The listing builds one solid part. Answer for the finished solid, in the listing's coordinates (mm). A direction names the side the tool comes from. Round coordinates to 2 decimals unless told otherwise and drop trailing zeros. Order: outer loops, then holes, each group sorted by start corner. A loop starts at its lowest first (then second) coordinate and runs counter-clockwise, first axis right, second up. Notation, with made-up numbers: (5.25, 35.5) - (56.25, 35.5) arc R13 cw to (56.25, 41.5) - close; hole circle Ø7 at (-7.75, 84). An arc over 180 degrees is marked (long way). Write item = value, one per line.
from build123d import *

# Parameters (mm, degrees)
ESQUISSE1_W             = 136.8
ESQUISSE1_H             = 11.8
BOSS_EXTRU_1_DEPTH      = 0.8
ESQUISSE2_W             = 136.8
ESQUISSE2_H             = 11.8
ESQUISSE2_W_2           = 135.2
ESQUISSE2_H_2           = 10.2
BOSS_EXTRU_2_DEPTH      = 1
ESQUISSE3_W             = 4
ESQUISSE3_H             = 0.8
BOSS_EXTRU_3_DEPTH      = 2
ESQUISSE4_W             = 11.8
ESQUISSE4_H             = 0.8
BOSS_EXTRU_4_DEPTH      = 5
ESQUISSE5_W             = 11.8
ESQUISSE5_H             = 0.8
BOSS_EXTRU_5_DEPTH      = 5
ESQUISSE6_R             = 1.2
ENL_V_MAT_EXTRU_1_DEPTH = 4
CONG_1_R                = 1


with BuildPart() as part:
    # Esquisse1 → Boss.-Extru.1 (new body)
    with BuildSketch(Plane(origin=(0, 0, 0), x_dir=(1, 0, 0), z_dir=(0, 1, 0))):
        with Locations((68.4, 5.9)):
            Rectangle(ESQUISSE1_W, ESQUISSE1_H)
    extrude(amount=BOSS_EXTRU_1_DEPTH)

    # Esquisse2 → Boss.-Extru.2 (add)
    with BuildSketch(Plane(origin=(0, 0.8, 0), x_dir=(1, 0, 0), z_dir=(0, 1, 0))):
        with Locations((68.4, 5.9)):
            Rectangle(ESQUISSE2_W, ESQUISSE2_H)
        with Locations((68.4, 5.9)):
            Rectangle(ESQUISSE2_W_2, ESQUISSE2_H_2, mode=Mode.SUBTRACT)
    extrude(amount=BOSS_EXTRU_2_DEPTH)

    # Esquisse3 → Boss.-Extru.3 (add)
    with BuildSketch(Plane(origin=(0, 1.8, 0), x_dir=(1, 0, 0), z_dir=(0, 1, 0))):
        Polygon((0.8, 3), (0, 3), (0, 0), (3, 0), (3, 0.8), (0.8, 0.8), align=None)
        Polygon((3, 11.8), (0, 11.8), (0, 8.8), (0.8, 8.8), (0.8, 11), (3, 11), align=None)
        Polygon((133.8, 11), (136, 11), (136, 8.8), (136.8, 8.8), (136.8, 11.8), (133.8, 11.8), align=None)
        with Locations((68.4, 11.4)):
            Rectangle(ESQUISSE3_W, ESQUISSE3_H)
        with Locations((68.4, 0.4)):
            Rectangle(ESQUISSE3_W, ESQUISSE3_H)
        Polygon((133.8, 0), (136.8, 0), (136.8, 3), (136, 3), (136, 0.8), (133.8, 0.8), align=None)
    extrude(amount=BOSS_EXTRU_3_DEPTH)

    # Esquisse4 → Boss.-Extru.4 (add)
    with BuildSketch(Plane(origin=(136.8, 0, 0), x_dir=(0, 0, -1), z_dir=(1, 0, 0))):
        with Locations((5.9, 0.4)):
            Rectangle(ESQUISSE4_W, ESQUISSE4_H)
    extrude(amount=BOSS_EXTRU_4_DEPTH)

    # Esquisse5 → Boss.-Extru.5 (add)
    with BuildSketch(Plane.ZY):
        with Locations((-5.9, 0.4)):
            Rectangle(ESQUISSE5_W, ESQUISSE5_H)
    extrude(amount=BOSS_EXTRU_5_DEPTH)

    # Esquisse6 → Enlèv. mat.-Extru.1 (cut)
    with BuildSketch(Plane.XZ):
        with Locations((140, -5.9)):
            Circle(ESQUISSE6_R)
        with Locations((-3.2, -5.9)):
            Circle(ESQUISSE6_R)
    extrude(amount=-ENL_V_MAT_EXTRU_1_DEPTH, mode=Mode.SUBTRACT)

    # Congé1
    cong_1_edges = [part.edges().sort_by_distance(p)[0] for p in [
        (141.8, 0.4, -11.8),
        (141.8, 0.4, 0),
        (-5, 0.4, -11.8),
        (-5, 0.4, 0),
        (0, 2.3, -11.8),
        (136.8, 2.3, -11.8),
        (136.8, 2.3, 0),
        (0, 2.3, 0),
    ]]
    fillet(cong_1_edges, radius=CONG_1_R)


solid = part.part
Q1. Determine the mould class of faces 5 (the face through (139.4, 0.8, -4.5)), 6 (the face through (69, 1, 0)), 7 (the face through (69, 2, -0.8)), 8 (the face through (138.8, 0.39, -5.85)) for opening direction Z: released by +Z, released by -Z, zero draft, split by the parting line, or undercut.
Model answer:
face_5 = zero draft
face_6 = released by +Z
face_7 = undercut
face_8 = undercut
Q2. Flat-ended cylindrical pins translate along their axes: P1, Ø0.9, axis at y = 3, z = -0.5, coming from the -X side; P2, Ø0.9, axis at x = 136.5, z = -5, coming from the +Y side; P3, Ø1.5, axis at y = 2.5, z = -2.5, coming from the +X side. Find the tip coordinate at first contact, or state that the pin passes through.
Model answer:
P1 = 0
P2 = 1.8
P3 = 136.8
Q3. Section A-A on z = -5.9 is taken. Determine the outline of the cut face in (x, y), then the cut area to 3 significant figures.
Model answer:
outline = (-5, 0) - (-4.4, 0) - (-4.4, 0.8) - (-5, 0.8) - close; (-2, 0) - (138.8, 0) - (138.8, 0.8) - (136.8, 0.8) - (136.8, 1.8) - (136, 1.8) - (136, 0.8) - (0.8, 0.8) - (0.8, 1.8) - (0, 1.8) - (0, 0.8) - (-2, 0.8) - close; (141.2, 0) - (141.8, 0) - (141.8, 0.8) - (141.2, 0.8) - close
area = 115 mm^2
Q4. For faces 1 (the face through (67, 2, -11)), 2 (the face through (-2.646, 0.394, -6.965)), 3 (the face through (0, 1.6, -6)), 4 (the face through (136.8, 1.6, -5.8)), determine the directions among +Z, -Z, +X, -X, +Y, -Y from which every point of the face is accessible in a straight line to the end or side of a thin tool.
Model answer:
face_1 = +Y
face_2 = +Y, -Y
face_3 = +Z, -Z, -X, +Y
face_4 = +Z, -Z, +X, +Y
Q5. Section B-B on x = 87 is taken. Determine the outline of the cut face in (y, z), then the cut area to 3 significant figures.
Model answer:
outline = (0, -11.8) - (1.8, -11.8) - (1.8, -11) - (0.8, -11) - (0.8, -0.8) - (1.8, -0.8) - (1.8, 0) - (0, 0) - close
area = 11.0 mm^2
Q6. Section C-C on y = 2.75 is taken. Count the separate pieces of the cut face and the enclosed holes in it, then the cut area to 3 significant figures.
Model answer:
separate_pieces = 6
enclosed_holes = 0
area = 22.2 mm^2
Q7. Find the intervals of material crossed by line 1 (Z direction, x = -3.2, y = 0.2); line 2 (X direction, y = 2.7, z = -10.5); line 3 (Z direction, x = 59, y = 1.75), in increasing order. Write a range as from..to.
Model answer:
line_1 = -11.8..-7.1, -4.7..0
line_2 = 0..0.8, 136..136.8
line_3 = -11.8..-11, -0.8..0
